Part model, mm, in its own coordinate system. A direction names the side the tool comes from. Give positions to 0.01 mm unless a question says otherwise; leave off trailing zeros. Write each loop counter-clockwise with the first axis right and the second up, starting at its lowest first coordinate (ties: lowest second). Pieces come first, ordered by that corner, then holes. Notation, with made-up numbers: M -27.5,74 L 25.5,74 A20 cw 25.5,103 Z; hole C 12,42 d7. An arc over 180 degrees is marked long. Answer as CSV lines item,"result". Start each with the question number.
Item 1: Pin check, flat tips, straight feed: pin 1 (2 mm diameter, centred on x = -6.5, z = -74, fed in from -Y); pin 2 (1 mm diameter, centred on x = 0, z = -46, fed in from -Y); pin 3 (6 mm diameter, centred on x = -11, z = -67, fed in from -Y). Stop position of each tip, or through.
Item 2: Band-saw the part on A-A, the plane z = -62.5. List the corners of the cut face in (x, y).
Item 3: Wall check: L1, parallel to Z at x = -12, y = -0.5; L2, parallel to X at y = -5, z = -32; L3, parallel to Y at x = -0.5, z = -95. Give the ranges that are in metal, low to high. Write a range as from..to.
Item 4: 3-axis set-ups, long thin cutter, end or side, ignore diameter. For faces 1 (the conical face through (9.02, -15.54, 7.35)), 2 (the cylindrical face through (2.17, -9.76, -69.62)): which of +Z, -Z, +X, -X, +Y, -Y reach the whole face in a straight line?
from build123d import *

# Parameters (mm, degrees)
BOSS_EXTRUDE1_DEPTH = 8
SKETCH2_OUTSIDE_W   = 87.056
SKETCH2_OUTSIDE_H   = 81.698
SKETCH2_OUTSIDE_R   = 17.320508076
CUT_EXTRUDE1_DEPTH  = 17
CUT_EXTRUDE1_TAPER  = 45
SKETCH3_R           = 10
BOSS_EXTRUDE2_DEPTH = 125


with BuildPart() as part:
    # Sketch1 → Boss-Extrude1 (new body, symmetric)
    with BuildSketch(Plane.XY):
        Polygon((-10, 17.320508076), (-20, 0), (-10, -17.320508076), (10, -17.320508076), (20, 0), (10, 17.320508076), align=None)
    extrude(amount=BOSS_EXTRUDE1_DEPTH, both=True)

    # Sketch2 outside → Cut-Extrude1 (cut, through all)
    with BuildSketch(Plane.XY.offset(8)):
        Rectangle(SKETCH2_OUTSIDE_W, SKETCH2_OUTSIDE_H)
        Circle(SKETCH2_OUTSIDE_R, mode=Mode.SUBTRACT)
    cut_extrude1 = extrude(amount=-CUT_EXTRUDE1_DEPTH, taper=CUT_EXTRUDE1_TAPER, mode=Mode.SUBTRACT)

    # Mirror1: Cut-Extrude1 across plane
    add(cut_extrude1.mirror(Plane.XY), mode=Mode.SUBTRACT)

    # Sketch3 → Boss-Extrude2 (add)
    with BuildSketch(Plane(origin=(0, 0, -8), x_dir=(-1, 0, 0), z_dir=(0, 0, -1))):
        Circle(SKETCH3_R)
    extrude(amount=BOSS_EXTRUDE2_DEPTH)


solid = part.part
Output:
1,pin 1,"y = -8.35"
1,pin 2,"y = -10"
1,pin 3,"y = -6"
2,outline,"C 0,0 d20"
3,L1,"-8..8"
3,L2,"-8.66..8.66"
3,L3,"-9.99..9.99"
4,face 1,"+Z, +X, -Y"
4,face 2,"-Z"
